from build123d import *

# Parameters (mm, degrees)
SKETCH1_R           = 0.6
SKETCH1_R_2         = 5
BOSS_EXTRUDE1_DEPTH = 10


with BuildPart() as part:
    # Sketch1 → Boss-Extrude1 (new body)
    with BuildSketch(Plane.XY):
        with BuildLine():
            Line((3.605551275, 6), (5, 6))
            ThreePointArc((5, 6), (5.707106781, 5.707106781), (6, 5))
            Line((6, 5), (6, 3.605551275))
            ThreePointArc((6, 3.605551275), (7, 0), (6, -3.605551275))
            Line((6, -3.605551275), (6, -5))
            ThreePointArc((6, -5), (5.707106781, -5.707106781), (5, -6))
            Line((5, -6), (3.605551275, -6))
            ThreePointArc((3.605551275, -6), (0, -7), (-3.605551275, -6))
            Line((-3.605551275, -6), (-5, -6))
            ThreePointArc((-5, -6), (-5.707106781, -5.707106781), (-6, -5))
            Line((-6, -5), (-6, -3.605551275))
            ThreePointArc((-6, -3.605551275), (-7, 0), (-6, 3.605551275))
            Line((-6, 3.605551275), (-6, 5))
            ThreePointArc((-6, 5), (-5.707106781, 5.707106781), (-5, 6))
            Line((-5, 6), (-3.605551275, 6))
            ThreePointArc((-3.605551275, 6), (0, 7), (3.605551275, 6))
        make_face()
        with Locations((5, 5)):
            Circle(SKETCH1_R, mode=Mode.SUBTRACT)
        with Locations(Location((-5, 5, 0), (0, 0, 180))):
            Circle(SKETCH1_R, mode=Mode.SUBTRACT)
        with Locations(Location((5, -5, 0), (0, 0, 180))):
            Circle(SKETCH1_R, mode=Mode.SUBTRACT)
        with Locations((-5, -5)):
            Circle(SKETCH1_R, mode=Mode.SUBTRACT)
        Circle(SKETCH1_R_2, mode=Mode.SUBTRACT)
    extrude(amount=BOSS_EXTRUDE1_DEPTH)


solid = part.part
Check sheet for the modelled part. Datum: model origin and axes. Units: mm. A direction names the side the tool comes from. Coordinates: 2 decimals unless noted, no trailing zeros. Loops run counter-clockwise (first coordinate to the right, second up) from the corner with the lowest first, then second, coordinate; pieces in that order, holes last. Notation, with made-up numbers: (20, 68.25) -> (76, 68.25) arc R10 cw to (76, 78.25) -> close; hole circle Ø4 at (13.5, 13). An arc over 180 degrees is marked (long way). Write item = value, one per line. Start each with the question number.
1. Section check C-C on y = 5.25. Record the cut outline in (x, z), then the cut area to 3 significant figures.
2. Depth check by flat-ended pin: P1, Ø3, axis at x = -4, z = 5, coming from the +Y side; P2, Ø1.1, axis at x = -4.5, z = 3.5, coming from the -Y side; P3, Ø0.7, axis at y = -4, z = 4.5, coming from the +X side; P4, Ø1.1, axis at x = 5, y = 5, coming from the -Z side. Enter the tip coordinate at first touch or a pass-through.
3. Section check A-A on x = 0. Record the cut outline in (y, z).
4. Tool access check on faces 1 (the flat face through (6, 4, 5)), 2 (the flat face through (4, -6, 5)), 3 (the flat face through (-6, -4, 5)). Record the directions out of +Z, -Z, +X, -X, +Y, -Y that give a thin tool (end or side, any length) a straight path to the whole face; none if there is none.
5. Draft check along X on faces 4 (the cylindrical face through (-1.08, -4.88, 4.93)), 5 (the cylindrical face through (5.699, 5.715, 4.93)), 6 (the cylindrical face through (5.476, -4.635, 4.93)), 7 (the cylindrical face through (-5.715, 5.699, 4.93)). Enter one of: released by +X, released by -X, zero draft, split by the parting line, or undercut.
6. Section check D-D on x = -2.5. Record the cut outline in (y, z).
7. Section check B-B on z = 2.25. Record the cut outline in (x, y), then the cut area to 3 significant figures.
8. Material ranges on line 1 (Y direction, x = 0, z = 4.5); line 2 (Y direction, x = 5.5, z = 7); line 3 (X direction, y = 3.5, z = 5), recorded low to high.
Responses:
q1.outline = (-5.97, 0) -> (-5.55, 0) -> (-5.55, 10) -> (-5.97, 10) -> close; (-4.45, 0) -> (4.45, 0) -> (4.45, 10) -> (-4.45, 10) -> close; (5.55, 0) -> (5.97, 0) -> (5.97, 10) -> (5.55, 10) -> close
q1.area = 97.5 mm2
q2.P1 = 6.54
q2.P2 = -6
q2.P3 = 6
q2.P4 = through
q3.outline = (-7, 0) -> (-5, 0) -> (-5, 10) -> (-7, 10) -> close; (5, 0) -> (7, 0) -> (7, 10) -> (5, 10) -> close
q4.face_1 = +Z, -Z, +X, +Y
q4.face_2 = +Z, -Z, +X, -Y
q4.face_3 = +Z, -Z, -X, -Y
q5.face_4 = undercut
q5.face_5 = released by +X
q5.face_6 = undercut
q5.face_7 = released by -X
q6.outline = (-6.54, 0) -> (-4.33, 0) -> (-4.33, 10) -> (-6.54, 10) -> close; (4.33, 0) -> (6.54, 0) -> (6.54, 10) -> (4.33, 10) -> close
q7.outline = (-6, -5) arc R1 ccw to (-5, -6) -> (-3.61, -6) arc R7 ccw to (3.61, -6) -> (5, -6) arc R1 ccw to (6, -5) -> (6, -3.61) arc R7 ccw to (6, 3.61) -> (6, 5) arc R1 ccw to (5, 6) -> (3.61, 6) arc R7 ccw to (-3.61, 6) -> (-5, 6) arc R1 ccw to (-6, 5) -> (-6, 3.61) arc R7 ccw to (-6, -3.61) -> close; hole circle Ø1.2 at (-5, -5); hole circle Ø1.2 at (-5, 5); hole circle Ø10 at (0, 0); hole circle Ø1.2 at (5, -5); hole circle Ø1.2 at (5, 5)
q7.area = 79.6 mm2
q8.line_1 = -7 to -5, 5 to 7
q8.line_2 = -5.87 to -5.33, -4.67 to 4.67, 5.33 to 5.87
q8.line_3 = -6.06 to -3.57, 3.57 to 6.06
